```python
from build123d import *

# Parameters (mm, degrees)
SKETCH2_W           = 13.0048
SKETCH2_H           = 8.9916
BOSS_EXTRUDE1_DEPTH = 4.0005
SKETCH4_R           = 2.7559
BOSS_EXTRUDE2_DEPTH = 16.51


with BuildPart() as part:
    # Sketch2 → Boss-Extrude1 (new body, symmetric)
    with BuildSketch(Plane.XY):
        with Locations((0, -4.4958)):
            Rectangle(SKETCH2_W, SKETCH2_H)
    extrude(amount=BOSS_EXTRUDE1_DEPTH, both=True)

    # Sketch3 → Revolve2 (revolve)
    with BuildSketch(Plane.XY):
        Polygon((-3.175, 10.0076), (-3.175, 2.0066), (-3.875, 2.0066), (-3.875, 0), (0, 0), (0, 10.0076), align=None)
    revolve(axis=Axis((0, 0, 0), (0, 1, 0)))

    # Sketch4 → Boss-Extrude2 (add)
    with BuildSketch(Plane(origin=(0, 10.0076, 0), x_dir=(1, 0, 0), z_dir=(0, 1, 0))):
        Circle(SKETCH4_R)
    extrude(amount=BOSS_EXTRUDE2_DEPTH)


solid = part.part
```
Verification items for the finished model (mm, model axes). A direction names the side the tool comes from. Round coordinates to 2 decimals unless told otherwise and drop trailing zeros. Order: outer loops, then holes, each group sorted by start corner. A loop starts at its lowest first (then second) coordinate and runs counter-clockwise, first axis right, second up.
1) Cross-section at C-C, the plane x = 5.25. Record the cut outline in (y, z), plus the area to 3 significant figures.
Geometry says:
outline: (-8.99, -4) - (0, -4) - (0, 4) - (-8.99, 4) - close
area: 71.9 mm2
2) Material ranges on line 1 (X direction, y = 25, z = 0); line 2 (Y direction, x = 2.25, z = -2.5); line 3 (Y direction, x = -5.5, z = -3), recorded low to high.
Geometry says:
line 1: x = -2.76 to 2.76
line 2: y = -8.99 to 2.01
line 3: y = -8.99 to 0
3) Tool access check on faces 1 (the cylindrical face through (0.69, 5.95, -3.1)), 2 (the flat face through (0, -8.992, 0)). Record the directions out of +Z, -Z, +X, -X, +Y, -Y that give a thin tool (end or side, any length) a straight path to the whole face; none if there is none.
Geometry says:
face 1: +Y
face 2: +Z, -Z, +X, -X, -Y
4) Depth check by flat-ended pin: pin 1 (3 mm diameter, centred on x = 4, z = 2, fed in from +Y); pin 2 (1 mm diameter, centred on x = 1.5, y = 18.5, fed in from +Z); pin 3 (1 mm diameter, centred on y = 8.5, z = 1, fed in from +X). Enter the tip coordinate at first touch or a pass-through.
Geometry says:
pin 1: stops at y = 10.01
pin 2: stops at z = 2.57
pin 3: stops at x = 3.14
5) Cross-section at A-A, the plane z = 0. Record the cut outline in (x, y) (3 decimals).
Geometry says:
outline: (-6.502, -8.992) - (6.502, -8.992) - (6.502, 0) - (3.875, 0) - (3.875, 2.007) - (3.175, 2.007) - (3.175, 10.008) - (2.756, 10.008) - (2.756, 26.518) - (-2.756, 26.518) - (-2.756, 10.008) - (-3.175, 10.008) - (-3.175, 2.007) - (-3.875, 2.007) - (-3.875, 0) - (-6.502, 0) - close
